Autodesk Inventor part; units mm, degrees
ref_plane "Work Plane1" through (0, 0, 15) normal (0, 0, 1) x (1, 0, 0)
ref_plane "YZ Plane" through (0, 0, 0) normal (1, 0, 0) x (0, 1, 0)
ref_plane "XZ Plane" through (0, 0, 0) normal (0, 1, 0) x (-1, 0, 0)
sketch "Sketch1" plane through (0, 0, 0) normal (0, 0, 1) x (1, 0, 0)
  line L0 (0, 0) -> (-140, 0)
  line L1 (0, 0) -> (0, 7)
  line L2 (-2, 9) -> (-115, 9)
  line L3 (-115, 9) -> (-115, 15)
  line L4 (-115, 15) -> (-125, 15)
  line L5 (-125, 15) -> (-125, 10)
  line L6 (-125, 10) -> (-138, 10)
  line L7 (-140, 8) -> (-140, 0)
  line L8 (-138, 10) -> (-140, 8)
  line L9 (-2, 9) -> (0, 7)
  line L10 (-267.7899, 0) -> (-197.3543, 0) construction
  point P0 (0, 9)
  point P1 (-140, 10)
  point P2 (-120, 15)
  dimension "d1" = 140
  dimension "d2" = 15
  dimension "d3" = 10
  dimension "d4" = 15
  dimension "d5" = 9
  dimension "d6" = 10
  dimension "d7" = 2
  dimension "d8" = 2
  dimension "d9" = 2
  dimension "d10" = 2
revolve "Revolution1" add sketch "Sketch1" angle 360 about axis through (-267.7899, 0, 0) along (1, 0, 0)
ref_plane "Work Plane1" through (0, 0, 15) normal (0, 0, 1) x (1, 0, 0)
sketch "Sketch2" plane through (0, 0, 15) normal (0, 0, 1) x (1, 0, 0)
  circle A0 centre (-120, 0) radius 3
  line L0 (-115, -15) -> (-115, 15)
  point P0 (0, 0)
  dimension "d13" = 6
  dimension "d14" = 5
extrude "Extrusion1" cut sketch "Sketch2" against normal blind 5
pattern_circular "Circular Pattern1" count 3 over 360 about axis through (-58.5, 0, 0) along (1, 0, 0) of "Extrusion1"
properties part number "Coluna do Ferramental"
Source: CAD feature listing. Evaluate the final solid. Frame: model axes, mm. A direction names the side the tool comes from. Round coordinates to 2 decimals unless told otherwise and drop trailing zeros. Loops run counter-clockwise (first coordinate to the right, second up) from the corner with the lowest first, then second, coordinate; pieces in that order, holes last. Notation, with made-up numbers: M -31.5,-11 L 1.5,-11 A33 ccw 1.5,26 Z; hole C 30.25,15.5 d7. An arc over 180 degrees is marked long. Return JSON: item names as keys, results as strings. Group by question number.
1. Section query D-D on z = 11.5. Output: boundary loops of the cut face in (x, y), and give its area (3 significant figures).
2. Material intervals for line 1 along X through (y, z) = (0, 11); line 2 along Y through (x, z) = (-120, 11.25); line 3 along Y through (x, z) = (-120, 12.9), sorted ascending. Write a range as from..to.
3. Section query C-C on x = -120. Output: boundary loops of the cut face in (y, z).
4. Section query A-A on z = 0. Output: boundary loops of the cut face in (x, y), and give its area (3 significant figures).
5. Mould query, pull axis X, two halves, no side actions, for faces 1 (the face through (-140, 0, 0)), 2 (the face through (-59.291, -1.172, -8.923)), 3 (the face through (-117.23, -10.28, -7.26)), 4 (the face through (-117.14, 0.9, 12.54)). Classes: released by +X, released by -X, zero draft, split by the parting line, or undercut.
6. Section query B-B on y = 0. Output: boundary loops of the cut face in (x, z), and give its area (3 significant figures).
7. Pin query (flat end, axial travel): pin 1 (1.5 mm diameter, centred on x = -29.5, y = -5.5, fed in from -Z); pin 2 (8 mm diameter, centred on x = -39, y = 11, fed in from -Z); pin 3 (12 mm diameter, centred on x = -84.5, z = -1, fed in from +Y). Return the tip coordinate at first contact, or that it passes through.
8. Reachability of faces 5 (the face through (0, 0, 0)), 6 (the face through (-120.042, -8.681, -4.964)), 7 (the face through (-125, 3, -10)), 8 (the face through (-115, 6.5, -6.5)), 9 (the face through (-120, 0, 10)) from +Z, -Z, +X, -X, +Y, -Y: full face, straight path, thin tool, end or side. Return the list, or none.
Checks:
{
 "1": {"outline": "M -125,-9.63 L -115,-9.63 L -115,9.63 L -125,9.63 Z; hole C -120,0 d6", "area": "164 mm²"},
 "2": {"line 1": "x = -125..-123, -117..-115", "line 2": "y = -9.92..-3, 3..9.92", "line 3": "y = -7.65..-3, 3..7.65"},
 "3": {"outline": "M -14.23,-4.75 L -10.16,-2.4 L -7.16,-7.6 L -11.23,-9.95 A15 ccw 11.23,-9.95 L 7.16,-7.6 L 10.16,-2.4 L 14.23,-4.75 A15 ccw 3,14.7 L 3,10 L -3,10 L -3,14.7 A15 ccw Z"},
 "4": {"outline": "M -140,-8 L -138,-10 L -125,-10 L -125,-15 L -115,-15 L -115,-9 L -2,-9 L 0,-7 L 0,7 L -2,9 L -115,9 L -115,15 L -125,15 L -125,10 L -138,10 L -140,8 Z", "area": "2,660 mm²"},
 "5": {"face 1": "released by -X", "face 2": "zero draft", "face 3": "undercut", "face 4": "undercut"},
 "6": {"outline": "M -140,-8 L -138,-10 L -125,-10 L -125,-15 L -115,-15 L -115,-9 L -2,-9 L 0,-7 L 0,7 L -2,9 L -115,9 L -115,15 L -117,15 L -117,10 L -123,10 L -123,15 L -125,15 L -125,10 L -138,10 L -140,8 Z", "area": "2,630 mm²"},
 "7": {"pin 1": "stops at z = -7.64", "pin 2": "stops at z = -5.66", "pin 3": "stops at y = 9"},
 "8": {"face 5": "+Z, -Z, +X, +Y, -Y", "face 6": "none", "face 7": "-X", "face 8": "+X", "face 9": "+Z"}
}
